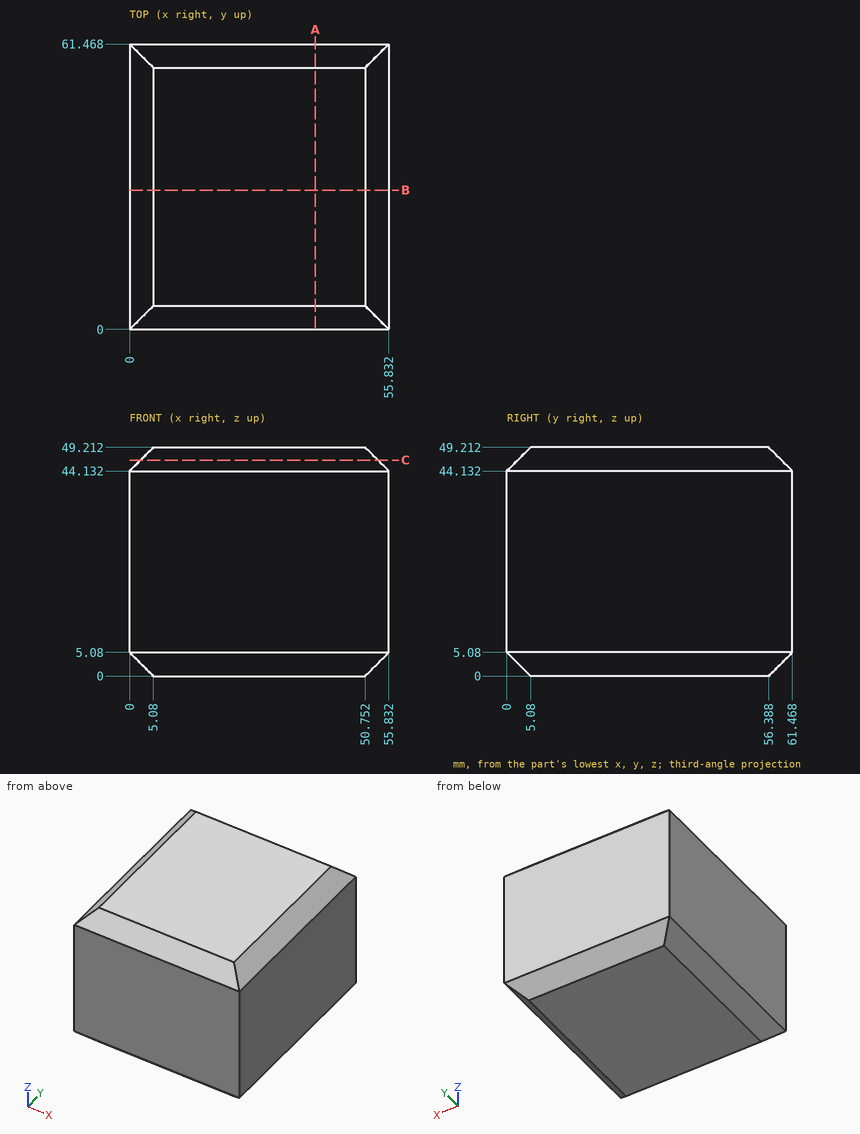
Input: dimensioned drawing with shaded views. Units: mm. Origin: part minimum x, y, z. Give positions to 0.01 mm unless a question says otherwise; leave off trailing zeros. Write each loop counter-clockwise with the first axis right and the second up, starting at its lowest first coordinate (ties: lowest second). Pieces come first, ordered by that corner, then holes. Notation, with made-up numbers: (22.5, 28) - (51.5, 28) arc R6 ccw to (51.5, 37) - close; hole circle Ø4 at (-29, -37). An arc over 180 degrees is marked (long way). Write item = value, one per line. Start each with the question number.
1) Material intervals for L1, parallel to Y at x = 12.5, z = 3; L2, parallel to Z at x = 3, y = 53; L3, parallel to Y at x = 40, z = 4.5, sorted ascending. Write a range as [from, to].
2) Cut plane A-A (x = 40). Return loops of the section in (y, z), and give its area (3 significant figures).
3) Cut plane B-B (y = 30). Return loops of the section in (x, z), and give its area (3 significant figures).
4) Cut plane C-C (z = 46.5). Return loops of the section in (x, y) (1 decimal), and give its area (3 significant figures).
Answers follow:
q1.L1 = [2.08, 59.39]
q1.L2 = [2.08, 47.13]
q1.L3 = [0.58, 60.89]
q2.outline = (0, 5.08) - (5.08, 0) - (56.39, 0) - (61.47, 5.08) - (61.47, 44.13) - (56.39, 49.21) - (5.08, 49.21) - (0, 44.13) - close
q2.area = 2,970 mm^2
q3.outline = (0, 5.08) - (5.08, 0) - (50.75, 0) - (55.83, 5.08) - (55.83, 44.13) - (50.75, 49.21) - (5.08, 49.21) - (0, 44.13) - close
q3.area = 2,700 mm^2
q4.outline = (2.4, 2.4) - (53.5, 2.4) - (53.5, 59.1) - (2.4, 59.1) - close
q4.area = 2,900 mm^2
